Can you work these out from the model? Positions are in its coordinate system, mm. A direction names the side the tool comes from. Round coordinates to 2 decimals unless told otherwise and drop trailing zeros. Order: outer loops, then holes, each group sorted by start corner. A loop starts at its lowest first (then second) coordinate and runs counter-clockwise, first axis right, second up. Notation, with made-up numbers: (31, 28) -> (43, 28) arc R21 ccw to (43, 67) -> close; hole circle Ø8 at (-25, -16.75). An arc over 180 degrees is marked (long way). Use a Markdown table: item, result. Add a question column.
Q1. For faces 1 (the face through (13, 0, 2)), 2 (the face through (13.439, 12.394, -3.131)), which set-ups out of +Z, -Z, +X, -X, +Y, -Y let a thin tool reach every point of the face, with its end or its side?
Q2. I need wall thicknesses on line 1 along Y through (x, z) = (12.7, -2.5); line 2 along Z through (x, y) = (4.75, 14.25) (3 decimals); line 3 along Y through (x, z) = (13.75, -4.5). Which ranges of each line are inside material? Lowest first, please. Write a range as [from, to].
Q3. If we section it at D-D on x = 17.75: List the corners of the cut face in (y, z) for me (3 decimals).
Q4. If we section it at B-B on x = 12.7: List the corners of the cut face in (y, z) for me (3 decimals).
Q5. If we section it at A-A on z = -4.25: List the corners of the cut face in (x, y) for me.
Q6. I'm going to push flat-ended pins straight in: pin 1 Ø3 at (x, y) = (22.5, 6.5) entering from -Z; pin 2 Ø4 at (y, z) = (10, -3) entering from -X. Where does each tip first touch, or does it pass through?
```python
from build123d import *

# Parameters (mm, degrees)
F0_W     = 25.4
F0_H     = 25.4
F0_R     = 2.3
F0_R_2   = 0.8
F1_DEPTH = 3.175
F2_DEPTH = 6.35


with BuildPart() as f1:
    # F0 (on Top) → F1 (new body)
    with BuildSketch(Plane.XY):
        with Locations((12.7, 12.7)):
            Rectangle(F0_W, F0_H)
        with Locations((12.7, 12.7)):
            Circle(F0_R, mode=Mode.SUBTRACT)
        with Locations((12.7, 12.7)):
            Circle(F0_R)
        with Locations((12.7, 12.7)):
            Circle(F0_R_2, mode=Mode.SUBTRACT)
        with Locations((12.7, 12.7)):
            Circle(F0_R_2)
    extrude(amount=F1_DEPTH)

    # F0 (on Top) → F2 (join)
    with BuildSketch(Plane.XY):
        with Locations((12.7, 12.7)):
            Circle(F0_R)
        with Locations((12.7, 12.7)):
            Circle(F0_R_2, mode=Mode.SUBTRACT)
    extrude(amount=-F2_DEPTH)


solid = f1.part
```
Answer below:
| question | item | result |
|---|---|---|
| 1 | face 1 | +Z, -Z, +X, -X, -Y |
| 1 | face 2 | -Z |
| 2 | line 1 | [10.4, 11.9], [13.5, 15] |
| 2 | line 2 | [0, 3.175] |
| 2 | line 3 | [10.65, 14.75] |
| 3 | outline | (0, 0) -> (25.4, 0) -> (25.4, 3.175) -> (0, 3.175) -> close |
| 4 | outline | (0, 0) -> (10.4, 0) -> (10.4, -6.35) -> (11.9, -6.35) -> (11.9, 0) -> (13.5, 0) -> (13.5, -6.35) -> (15, -6.35) -> (15, 0) -> (25.4, 0) -> (25.4, 3.175) -> (0, 3.175) -> close |
| 5 | outline | circle Ø4.6 at (12.7, 12.7); hole circle Ø1.6 at (12.7, 12.7) |
| 6 | pin 1 | z = 0 |
| 6 | pin 2 | x = 10.51 |
